Check sheet for the modelled part. Datum: model origin and axes. Units: mm. A direction names the side the tool comes from. Coordinates: 2 decimals unless noted, no trailing zeros. Loops run counter-clockwise (first coordinate to the right, second up) from the corner with the lowest first, then second, coordinate; pieces in that order, holes last. Notation, with made-up numbers: M 27,45 L 66,45 A9 cw 66,58 Z; hole C -3.5,84.5 d3. An arc over 180 degrees is marked long. Return JSON: item names as keys, results as strings.
from build123d import *

# Parameters (mm, degrees)
EXTRUSION1_DEPTH             = 48
ENL_V_MAT_EXTRU_1_DEPTH      = 97
R_P_TITION_CIRCULAIRE1_COUNT = 2
R_P_TITION_CIRCULAIRE1_ANGLE = 90


with BuildPart() as part:
    # Esquisse1 → Extrusion1 (new body, symmetric)
    with BuildSketch(Plane.XY):
        with BuildLine():
            Line((-6, 5), (-6, -5))
            ThreePointArc((-6, -5), (-5.707106781, -5.707106781), (-5, -6))
            Line((-5, -6), (5, -6))
            ThreePointArc((5, -6), (5.707106781, -5.707106781), (6, -5))
            Line((6, -5), (6, 5))
            ThreePointArc((6, 5), (5.707106781, 5.707106781), (5, 6))
            Line((5, 6), (-5, 6))
            ThreePointArc((-5, 6), (-5.707106781, 5.707106781), (-6, 5))
        make_face()
    extrude(amount=EXTRUSION1_DEPTH, both=True)

    # Esquisse3 → Enl_v. mat.-Extru.1 (cut, through all)
    with BuildSketch(Plane.XY.offset(48)):
        Polygon((6, 2), (4.8, 2), (4.8, 4), (2, 1), (2, -1), (4.8, -4), (4.8, -2), (6, -2), align=None)
    enl_v_mat_extru_1 = extrude(amount=-ENL_V_MAT_EXTRU_1_DEPTH, mode=Mode.SUBTRACT)

    # R_p_tition circulaire1: Enl_v. mat.-Extru.1 ×2 about axis
    r_p_tition_circulaire1_axis = Axis((0, 0, 0), (0, 0, 1))
    for i in range(1, R_P_TITION_CIRCULAIRE1_COUNT):
        add(enl_v_mat_extru_1.rotate(r_p_tition_circulaire1_axis, i * R_P_TITION_CIRCULAIRE1_ANGLE / (R_P_TITION_CIRCULAIRE1_COUNT - 1)), mode=Mode.SUBTRACT)


solid = part.part
1) Draft check along X on faces 1 (the face through (2.5, 3.4, 0.7)), 2 (the face through (-6, 0, 1)), 3 (the face through (-3, 6, 1)), 4 (the face through (2, 0, 1)). Enter one of: +X half, -X half, draft (parallel to the pull), parting line (faces both ways), or undercut.
Answers:
{"face 1": "undercut", "face 2": "-X half", "face 3": "draft", "face 4": "+X half"}
2) Section check A-A on y = 3. Record the cut outline in (x, z), then the cut area to 3 significant figures.
Answers:
{"outline": "M -6,-48 L -2.07,-48 L -2.07,48 L -6,48 Z; M 2.07,-48 L 3.87,-48 L 3.87,48 L 2.07,48 Z; M 4.8,-48 L 6,-48 L 6,48 L 4.8,48 Z", "area": "665 mm²"}
3) Set-up check for faces 5 (the face through (0, 2, 1)), 6 (the face through (-1, -1, -48)): record each of +Z, -Z, +X, -X, +Y, -Y from which the full face is reachable in a straight line by a thin tool's end or side.
Answers:
{"face 5": "+Z, -Z, +Y", "face 6": "-Z, +X, -X, +Y, -Y"}
4) Go/stop test with flat-tipped pins: pin 1 Ø0.6 at (x, z) = (5.5, -20.5) entering from -Y; pin 2 Ø1.6 at (y, z) = (-0.5, 1.5) entering from +X. Record where each tip stops, or that it passes through.
Answers:
{"pin 1": "y = -5.98", "pin 2": "x = 2.28"}
5) Section check B-B on z = 3.5. Record the cut outline in (x, y).
Answers:
{"outline": "M -6,-5 A1 ccw -5,-6 L 5,-6 A1 ccw 6,-5 L 6,-2 L 4.8,-2 L 4.8,-4 L 2,-1 L 2,1 L 4.8,4 L 4.8,2 L 6,2 L 6,5 A1 ccw 5,6 L 2,6 L 2,4.8 L 4,4.8 L 1,2 L -1,2 L -4,4.8 L -2,4.8 L -2,6 L -5,6 A1 ccw -6,5 Z"}
6) Scan lines: line 1 along X through (y, z) = (3.25, 8); line 2 along X through (y, z) = (5, 14); line 3 along Y through (x, z) = (3, 32). Record each from-to range of solid material in increasing order. Write a range as [from, to].
Answers:
{"line 1": "[-6, -2.34], [2.34, 4.1], [4.8, 6]", "line 2": "[-6, -2], [2, 6]", "line 3": "[-6, -2.07], [2.07, 3.87], [4.8, 6]"}
